```python
from build123d import *

# Parameters (mm, degrees)
BOSS_EXTRUDE1_DEPTH = 10
SKETCH2_W           = 60
SKETCH2_H           = 5
BOSS_EXTRUDE2_DEPTH = 25
FILLET1_R           = 5
SKETCH3_R           = 1.75
CUT_EXTRUDE1_DEPTH  = 25
SKETCH4_R           = 1.75
CUT_EXTRUDE2_DEPTH  = 25
CUT_EXTRUDE3_DEPTH  = 25
SKETCH6_W           = 7
SKETCH6_H           = 40
BOSS_EXTRUDE3_DEPTH = 45
SKETCH7_R           = 11.5
SKETCH7_R_2         = 1.75
CUT_EXTRUDE4_DEPTH  = 45


with BuildPart() as part:
    # Sketch1 → Boss-Extrude1 (new body)
    with BuildSketch(Plane.XY):
        with BuildLine():
            Line((60, 35), (0, 35))
            Line((0, 35), (0, 40))
            ThreePointArc((0, 40), (-7.071067812, 37.071067812), (-10, 30))
            Line((-10, 30), (-10, 10))
            ThreePointArc((-10, 10), (-7.071067812, 2.928932188), (0, 0))
            Line((0, 0), (60, 0))
            ThreePointArc((60, 0), (67.071067812, 2.928932188), (70, 10))
            Line((70, 10), (70, 30))
            ThreePointArc((70, 30), (67.071067812, 37.071067812), (60, 40))
            Line((60, 40), (60, 35))
        make_face()
    extrude(amount=BOSS_EXTRUDE1_DEPTH)

    # Sketch2 → Boss-Extrude2 (add)
    with BuildSketch(Plane.XY.offset(10)):
        with Locations((30, 37.5)):
            Rectangle(SKETCH2_W, SKETCH2_H)
    extrude(amount=-BOSS_EXTRUDE2_DEPTH)

    # Fillet1
    fillet1_edges = [part.edges().sort_by_distance(p)[0] for p in [
        (0, 37.5, -15),
        (60, 37.5, -15),
    ]]
    fillet(fillet1_edges, radius=FILLET1_R)

    # Sketch3 → Cut-Extrude1 (cut)
    with BuildSketch(Plane.XY.offset(10)):
        with Locations((0, 6)):
            Circle(SKETCH3_R)
        with Locations((60, 6)):
            Circle(SKETCH3_R)
    extrude(amount=-CUT_EXTRUDE1_DEPTH, mode=Mode.SUBTRACT)

    # Sketch4 → Cut-Extrude2 (cut)
    with BuildSketch(Plane(origin=(0, 35, 0), x_dir=(-1, 0, 0), z_dir=(0, -1, 0))):
        with Locations((-55, 7.5)):
            Circle(SKETCH4_R)
        with Locations((-30, 7.5)):
            Circle(SKETCH4_R)
        with Locations((-5, 7.5)):
            Circle(SKETCH4_R)
    extrude(amount=-CUT_EXTRUDE2_DEPTH, mode=Mode.SUBTRACT)

    # Sketch5 → Cut-Extrude3 (cut)
    with BuildSketch(Plane.XZ.offset(-35)):
        with BuildLine():
            Line((5, -14.75), (55, -14.75))
            ThreePointArc((55, -14.75), (58.358757211, -13.358757211), (59.75, -10))
            Line((59.75, -10), (59.75, -0.25))
            Line((59.75, -0.25), (59.75, 0))
            Line((59.75, 0), (60, 0))
            Line((60, 0), (60, -10))
            ThreePointArc((60, -10), (58.535533906, -13.535533906), (55, -15))
            Line((55, -15), (5, -15))
            ThreePointArc((5, -15), (1.464466094, -13.535533906), (0, -10))
            Line((0, -10), (0, 0))
            Line((0, 0), (0.25, 0))
            Line((0.25, 0), (0.25, -0.25))
            Line((0.25, -0.25), (0.25, -10))
            ThreePointArc((0.25, -10), (1.641242789, -13.358757211), (5, -14.75))
        make_face()
    extrude(amount=-CUT_EXTRUDE3_DEPTH, mode=Mode.SUBTRACT)

    # Sketch6 → Boss-Extrude3 (add)
    with BuildSketch(Plane.XY.offset(10)):
        with Locations((30, 20)):
            Rectangle(SKETCH6_W, SKETCH6_H)
    extrude(amount=BOSS_EXTRUDE3_DEPTH)

    # Sketch7 → Cut-Extrude4 (cut)
    with BuildSketch(Plane(origin=(33.5, 0, 0), x_dir=(0, 0, -1), z_dir=(1, 0, 0))):
        with Locations((-34, 20)):
            Circle(SKETCH7_R)
        with Locations((-49.5, 35.5)):
            Circle(SKETCH7_R_2)
        with Locations((-18.5, 35.5)):
            Circle(SKETCH7_R_2)
        with Locations((-18.5, 4.5)):
            Circle(SKETCH7_R_2)
        with Locations((-49.5, 4.5)):
            Circle(SKETCH7_R_2)
    extrude(amount=-CUT_EXTRUDE4_DEPTH, mode=Mode.SUBTRACT)


solid = part.part
```
Source: CAD feature listing. Evaluate the final solid. Frame: model axes, mm. A direction names the side the tool comes from. Coordinates: 2 decimals unless noted, no trailing zeros. Loops run counter-clockwise (first coordinate to the right, second up) from the corner with the lowest first, then second, coordinate; pieces in that order, holes last. Notation, with made-up numbers: (38, 52.5) - (66, 52.5) arc R31 cw to (66, 86.5) - close; hole circle Ø11 at (-33.5, 64.25). An arc over 180 degrees is marked (long way). Answer as CSV lines item,"result".
1. Ray query, line 1 (Y direction, x = 0, z = 4.75); line 2 (Z direction, x = 19, y = 35.5); line 3 (Z direction, x = 49.5, y = 4.5). Return the intervals inside material, ascending.
Established:
line 1,"y = 0 to 4.25, 7.75 to 40"
line 2,"z = -14.75 to 10"
line 3,"z = 0 to 10"
2. Section A-A (z = -7.5). Return loops of the section in (x, y).
Established:
outline,"(0.25, 35) - (3.25, 35) - (3.25, 40) - (0.25, 40) - close; (6.75, 35) - (28.25, 35) - (28.25, 40) - (6.75, 40) - close; (31.75, 35) - (53.25, 35) - (53.25, 40) - (31.75, 40) - close; (56.75, 35) - (59.75, 35) - (59.75, 40) - (56.75, 40) - close"
3. Contact query for flat-ended pins moving along their axis: pin 1 (1 mm diameter, centred on x = 28, y = 29.5, fed in from -Z); pin 2 (4 mm diameter, centred on x = 40.5, z = -6.5, fed in from -Y); pin 3 (4.5 mm diameter, centred on y = 4.5, z = 18.5, fed in from +X). Output: stop coordinate, or through.
Established:
pin 1,"stops at z = 0"
pin 2,"stops at y = 35"
pin 3,"stops at x = 33.5"
4. Reachability of faces 4 (the cylindrical face through (30.05, 34.44, 19.89)), 5 (the flat face through (59.75, 37, -5)) from +Z, -Z, +X, -X, +Y, -Y: full face, straight path, thin tool, end or side. Return the list, or none.
Established:
face 4,"+X, -X"
face 5,"-Z, +X, +Y, -Y"
5. Section B-B (x = 29.5). Return loops of the section in (y, z).
Established:
outline,"(0, 0) - (35, 0) - (35, -5.82) - (40, -5.82) - (40, 55) - (0, 55) - close; (35, -14.75) - (40, -14.75) - (40, -9.18) - (35, -9.18) - close; hole circle Ø3.5 at (4.5, 18.5); hole circle Ø3.5 at (4.5, 49.5); hole circle Ø23 at (20, 34); hole circle Ø3.5 at (35.5, 18.5); hole circle Ø3.5 at (35.5, 49.5)"
6. Mould query, pull axis Z, two halves, no side actions, for faces 1 (the flat face through (51, 20, 10)), 2 (the flat face through (30, 37, -14.75)), 3 (the cylindrical face through (5.38, 37.47, -5.79)). Classes: released by +Z, released by -Z, zero draft, split by the parting line, or undercut.
Established:
face 1,"released by +Z"
face 2,"released by -Z"
face 3,"undercut"
7. Section D-D (y = 28.5). Return loops of the section in (x, z), then the cut area to 3 significant figures.
Established:
outline,"(-10, 0) - (70, 0) - (70, 10) - (33.5, 10) - (33.5, 26.25) - (26.5, 26.25) - (26.5, 10) - (-10, 10) - close; (26.5, 41.75) - (33.5, 41.75) - (33.5, 55) - (26.5, 55) - close"
area,"1,010 mm2"
8. Section C-C (z = 49.5). Return loops of the section in (x, y), then the cut area to 3 significant figures.
Established:
outline,"(26.5, 0) - (33.5, 0) - (33.5, 2.75) - (26.5, 2.75) - close; (26.5, 6.25) - (33.5, 6.25) - (33.5, 33.75) - (26.5, 33.75) - close; (26.5, 37.25) - (33.5, 37.25) - (33.5, 40) - (26.5, 40) - close"
area,"231 mm2"
